Could you check a few things on this drawing? It's one solid part, dimensions in mm from its lowest x, y, z. Coordinates: 2 decimals unless noted, no trailing zeros. Loops run counter-clockwise (first coordinate to the right, second up) from the corner with the lowest first, then second, coordinate; pieces in that order, holes last.
1) Imagine slicing it at B-B on z = 0.75. Please give me the cut outline in (x, y) (3 decimals).
2) If I drill on line 1 along X through (y, z) = (11, 1.95) (1 decimal); line 2 along X through (y, z) = (19.5, 2.3) (1 decimal); line 3 along Y through (x, z) = (57.5, 3.1), over which ranges is the centre line in solid material (lowest first)?
3) Imagine slicing it at A-A on y = 13. Please give me the cut outline in (x, z) (1 decimal), plus the area to 3 significant figures.
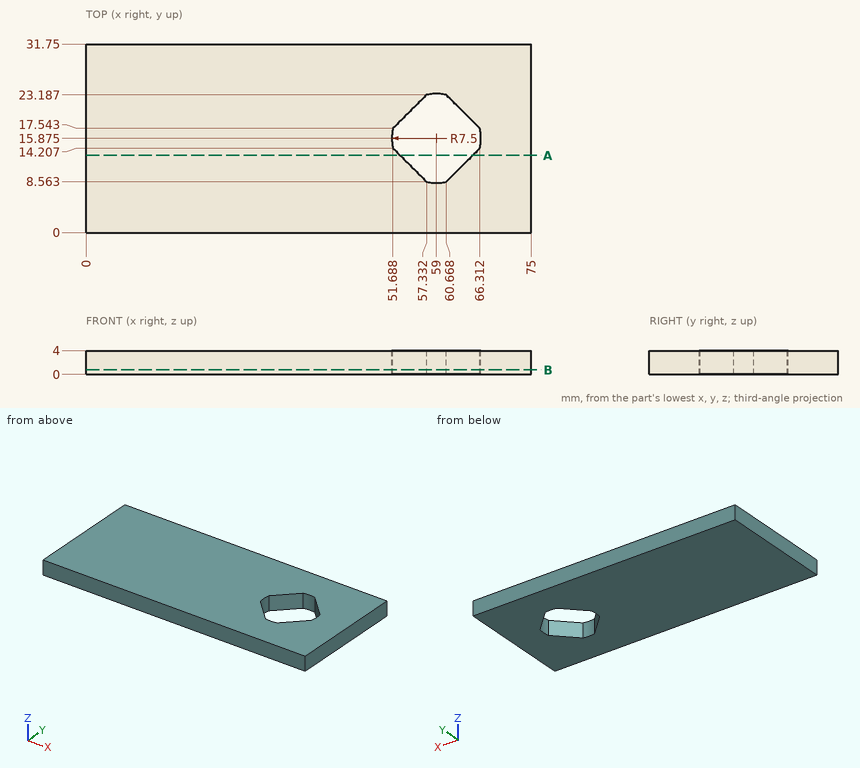
Filled in:
1. outline: (0, 0) - (75, 0) - (75, 31.75) - (0, 31.75) - close; hole (51.688, 14.207) - (57.332, 8.563) arc R7.5 ccw to (60.668, 8.563) - (66.312, 14.207) arc R7.5 ccw to (66.312, 17.543) - (60.668, 23.187) arc R7.5 ccw to (57.332, 23.187) - (51.688, 17.543) arc R7.5 ccw to start
2. line 1: x = 0 to 54.9, 63.1 to 75
2. line 2: x = 0 to 53.6, 64.4 to 75
2. line 3: y = 0 to 8.53, 23.22 to 31.75
3. outline: (0, 0) - (52.9, 0) - (52.9, 4) - (0, 4) - close; (65.1, 0) - (75, 0) - (75, 4) - (65.1, 4) - close
3. area: 251 mm2
